Autodesk Inventor part; units mm, degrees
ref_plane "YZ Plane" through (0, 0, 0) normal (1, 0, 0) x (0, 1, 0)
ref_plane "XZ Plane" through (0, 0, 0) normal (0, 1, 0) x (-1, 0, 0)
ref_plane "XY Plane" through (0, 0, 0) normal (0, 0, 1) x (1, 0, 0)
sketch "Skizze2" plane through (0, 0, 0) normal (0, 0, 1) x (1, 0, 0)
  line L0 (0, 14) -> (0, -14) construction
  line L1 (-14, 0) -> (14, 0) construction
  circle A0 centre (0, 0) radius 10
  dimension "d0" = 20
extrude "Grundkörper" add sketch "Skizze2" along normal blind 20
sketch "Skizze3" plane through (0, 0, 0) normal (0, 0, -1) x (-1, 0, 0)
  line L0 (0, -14) -> (0, 14)
  line L1 (-14, 0) -> (14, 0)
  point P0 (0, 0)
  point P1 (0, 0)
hole "12H7_Passbohrung" at (0, 0, 0) direction (0, 0, 1) diameter 12 depth 10
sketch "Skizze4" plane through (0, 0, 20) normal (0, 0, 1) x (1, 0, 0)
  line L0 (0, 14) -> (0, -14) construction
  line L1 (-14, 0) -> (14, 0) construction
  point P0 (0, 0)
  point P1 (0, 0)
hole "DIN7984_M5_Bohrung" at (0, 0, 20) direction (0, 0, -1) diameter 5.5 end through all counterbore diameter 10 counterbore depth 3.9
chamfer "Fase_Deckel" distance 3 angle 45 1 edges at (-10, 0, 20)
chamfer "Fase_Allgemein" distance 0.5 angle 45 2 edges at (0, -6, 0) (-10, 0, 0)
properties part number "200-60-DIFFERENTIAL-CONNECTOR-03" material "Edelstahl"
The listing builds one solid part. Answer for the finished solid, in the listing's coordinates (mm). A direction names the side the tool comes from. Coordinates: 2 decimals unless noted, no trailing zeros. Loops run counter-clockwise (first coordinate to the right, second up) from the corner with the lowest first, then second, coordinate; pieces in that order, holes last. Notation, with made-up numbers: (85.5, 10.5) - (120.5, 10.5) arc R22 ccw to (120.5, 23.5) - close; hole circle Ø6 at (-38, 72). An arc over 180 degrees is marked (long way). Use a Markdown table: item, result. Add a question column.
1) Find the intervals of material crossed by line 1 (Y direction, x = 0, z = 12.75); line 2 (Y direction, x = 0, z = 16.75); line 3 (Z direction, x = 2.75, y = 3.5), in increasing order.
2) The part is cut by section D-D, the plane z = 15. Give the vertices of the cut face in (x, y), and give its area (3 significant figures).
3) The part is cut by section C-C, the plane z = 8.75. Give the vertices of the cut face in (x, y), and give its area (3 significant figures).
4) For faces 4 (the cylindrical face through (0, -6, 5)), 5 (the cylindrical face through (2.685, 0.596, 13.007)), 6 (the flat face through (2.2, -2.2, 16.1)), determine the directions among +Z, -Z, +X, -X, +Y, -Y from which every point of the face is accessible in a straight line to the end or side of a thin tool.
5) Given pin 1 (1 mm diameter, centred on x = -8, z = 12.5, fed in from -Y); pin 2 (9 mm diameter, centred on x = 0, y = 0, fed in from +Z); pin 3 (6 mm diameter, centred on x = 3.5, z = 12, fed in from -Y), each flat-ended and moving along its own axis, determine where each tip first touches the part or whether it passes through.
6) The mould has two halves that part along Y. Classify faces 1 (the cylindrical face through (-2.17, 9.76, 8.63)), 2 (the flat face through (1, 3, 10)), 3 (the flat face through (4, -6, 0)): released by +Y, released by -Y, zero draft, split by the parting line, or undercut.
7) The part is cut by section A-A, the plane x = 0. Give the vertices of the cut face in (y, z).
Here are the results:
| question | item | result |
|---|---|---|
| 1 | line 1 | y = -10 to -2.75, 2.75 to 10 |
| 1 | line 2 | y = -10 to -5, 5 to 10 |
| 1 | line 3 | z = 10 to 16.1 |
| 2 | outline | circle Ø20 at (0, 0); hole circle Ø5.5 at (0, 0) |
| 2 | area | 290 mm^2 |
| 3 | outline | circle Ø20 at (0, 0); hole circle Ø12 at (0, 0) |
| 3 | area | 201 mm^2 |
| 4 | face 4 | -Z |
| 4 | face 5 | +Z, -Z |
| 4 | face 6 | +Z |
| 5 | pin 1 | stops at y = -6.61 |
| 5 | pin 2 | stops at z = 16.1 |
| 5 | pin 3 | stops at y = -9.99 |
| 6 | face 1 | split by the parting line |
| 6 | face 2 | undercut |
| 6 | face 3 | zero draft |
| 7 | outline | (-10, 0.5) - (-9.5, 0) - (-6.5, 0) - (-6, 0.5) - (-6, 10) - (-2.75, 10) - (-2.75, 16.1) - (-5, 16.1) - (-5, 20) - (-7, 20) - (-10, 17) - close; (2.75, 10) - (6, 10) - (6, 0.5) - (6.5, 0) - (9.5, 0) - (10, 0.5) - (10, 17) - (7, 20) - (5, 20) - (5, 16.1) - (2.75, 16.1) - close |
